from build123d import *

# Parameters (mm, degrees)
SKETCH1_W           = 45
SKETCH1_H           = 47
BOSS_EXTRUDE1_DEPTH = 2
SKETCH2_W           = 45
SKETCH2_H           = 2
BOSS_EXTRUDE2_DEPTH = 19.5
FILLET1_R           = 2
FILLET2_R           = 5
SKETCH3_W           = 25
SKETCH3_H           = 22.5
CUT_EXTRUDE1_DEPTH  = 39.99679474
SKETCH4_R           = 1.5
CUT_EXTRUDE2_DEPTH  = 54.958317246


with BuildPart() as part:
    # Sketch1 → Boss-Extrude1 (new body)
    with BuildSketch(Plane.XY):
        Rectangle(SKETCH1_W, SKETCH1_H)
    extrude(amount=BOSS_EXTRUDE1_DEPTH)

    # Sketch2 → Boss-Extrude2 (add)
    with BuildSketch(Plane(origin=(0, 0, 0), x_dir=(-1, 0, 0), z_dir=(0, 0, -1))):
        with Locations((0, -22.5)):
            Rectangle(SKETCH2_W, SKETCH2_H)
    extrude(amount=BOSS_EXTRUDE2_DEPTH)

    # Fillet1
    fillet1_edges = [part.edges().sort_by_distance(p)[0] for p in [
        (0, -23.5, 2),
    ]]
    fillet(fillet1_edges, radius=FILLET1_R)

    # Fillet2
    fillet2_edges = [part.edges().sort_by_distance(p)[0] for p in [
        (22.5, -22.5, -19.5),
        (-22.5, -22.5, -19.5),
    ]]
    fillet(fillet2_edges, radius=FILLET2_R)

    # Sketch3 → Cut-Extrude1 (cut, through all)
    with BuildSketch(Plane.XY.offset(2)):
        with Locations((0, 12.25)):
            Rectangle(SKETCH3_W, SKETCH3_H)
    extrude(amount=-CUT_EXTRUDE1_DEPTH, mode=Mode.SUBTRACT)

    # Sketch4 → Cut-Extrude2 (cut, through all)
    with BuildSketch(Plane(origin=(0, -21.5, 0), x_dir=(1, 0, 0), z_dir=(0, 1, 0))):
        with Locations(Location((0, 14.5, 0), (0, 0, 180))):
            Circle(SKETCH4_R)
    extrude(amount=-CUT_EXTRUDE2_DEPTH, mode=Mode.SUBTRACT)


solid = part.part
For this review, take the finished solid that the model builds, in its own axes (mm). A direction names the side the tool comes from. Give positions to 0.01 mm unless a question says otherwise; leave off trailing zeros. Order: outer loops, then holes, each group sorted by start corner. A loop starts at its lowest first (then second) coordinate and runs counter-clockwise, first axis right, second up. Notation, with made-up numbers: M 20,88.5 L 48,88.5 A14 ccw 48,114.5 Z; hole C 51,43 d10. An arc over 180 degrees is marked long. Answer in a Markdown table with one row per item. Add a question column.
(1) For pin 1 (6 mm diameter, centred on y = 11, z = -5, fed in from -X); pin 2 (1 mm diameter, centred on x = -3.5, z = -7.5, fed in from +Y); pin 3 (0.6 mm diameter, centred on x = 2, z = 0.5, fed in from +Y); pin 4 (12 mm diameter, centred on x = -3, y = -2, fed in from -Z), all flat-tipped, find the tip position at first contact; note any pin that passes through.
(2) Consider section C-C on x = -14.5. State the section outline as (y, z) points.
(3) Consider section B-B on y = 7. State the section outline as (x, z) points.
(4) For faces 4 (the face through (-21, -22.49, -18.07)), 5 (the face through (0, 1, 1)), 6 (the face through (0, -21.5, -10)), list the 3-axis set-ups (+Z, -Z, +X, -X, +Y, -Y) from which the entire face can be reached by the end or side of a thin tool; tool diameter is ignored.
(5) Mouldability with a two-part tool opening along X and no side actions: class faces 1 (the face through (-12.5, 12, 1)), 2 (the face through (-22.5, -5, 1)), 3 (the face through (0.32, -22.93, 1.4)) as +X half, -X half, draft (parallel to the pull), parting line (faces both ways), or undercut.
(6) Wall thickness on probe 1 along Y at (x, z) = (0, -3); probe 2 along Z at (x, y) = (-20, -13); probe 3 along Z at (x, y) = (0, -22.05): over which ranges is each line inside the solid? List them lowest first. Write a range as [from, to].
(7) Consider section D-D on y = -6.5. State the section outline as (x, z) points, and give its area (3 significant figures).
(8) Consider section A-A on x = 0. State the section outline as (y, z) points.
Evaluation:
| question | item | result |
|---|---|---|
| 1 | pin 1 | passes through |
| 1 | pin 2 | stops at y = -21.5 |
| 1 | pin 3 | stops at y = 1 |
| 1 | pin 4 | stops at z = 0 |
| 2 | outline | M -23.5,-19.5 L -21.5,-19.5 L -21.5,0 L 23.5,0 L 23.5,2 L -21.5,2 A2 ccw -23.5,0 Z |
| 3 | outline | M -22.5,0 L -12.5,0 L -12.5,2 L -22.5,2 Z; M 12.5,0 L 22.5,0 L 22.5,2 L 12.5,2 Z |
| 4 | face 4 | -Z, -X, +Y, -Y |
| 4 | face 5 | +Z, -Z, +Y |
| 4 | face 6 | -Z, +X, -X, +Y |
| 5 | face 1 | undercut |
| 5 | face 2 | -X half |
| 5 | face 3 | draft |
| 6 | probe 1 | y = [-23.5, -21.5] |
| 6 | probe 2 | z = [0, 2] |
| 6 | probe 3 | z = [-19.5, -16], [-13, 1.92] |
| 7 | outline | M -22.5,0 L 22.5,0 L 22.5,2 L -22.5,2 Z |
| 7 | area | 90.0 mm^2 |
| 8 | outline | M -23.5,-19.5 L -21.5,-19.5 L -21.5,-16 L -23.5,-16 Z; M -23.5,-13 L -21.5,-13 L -21.5,0 L 1,0 L 1,2 L -21.5,2 A2 ccw -23.5,0 Z |
